Model file for the job. Use its own axes, mm. Face numbers are marked on the shaded views. A direction names the side the tool comes from. Round coordinates to 2 decimals unless told otherwise and drop trailing zeros. Write each loop counter-clockwise with the first axis right and the second up, starting at its lowest first coordinate (ties: lowest second). Pieces come first, ordered by that corner, then holes.
```python
from build123d import *

# Parameters (mm, degrees)
SKETCH1_W           = 7
SKETCH1_H           = 1
BOSS_EXTRUDE1_DEPTH = 3


with BuildPart() as part:
    # Sketch1 → Boss-Extrude1 (new body, symmetric)
    with BuildSketch(Plane(origin=(0, 0, 0), x_dir=(1, 0, 0), z_dir=(0, 1, 0))):
        with Locations((-3.5, 0)):
            Rectangle(SKETCH1_W, SKETCH1_H)
        Polygon((1, 0.5), (0, 0.5), (0, -0.5), (0, -4), (10, -4), (10, -3), (1, -3), align=None)
    extrude(amount=BOSS_EXTRUDE1_DEPTH, both=True)


solid = part.part
```
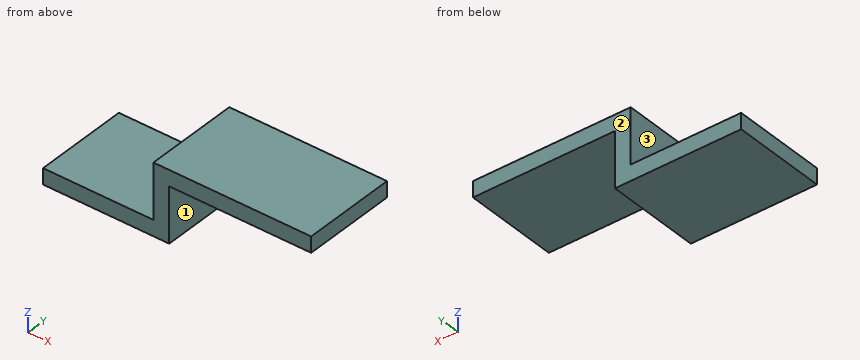
1) Cut at C-C on x = 2.5. List the corners of the cut face in (y, z), and give its area (3 significant figures).
2) Cut at A-A on y = 1.2. List the corners of the cut face in (x, z).
3) Which spindle directions (+Z, -Z, +X, -X, +Y, -Y) get a long thin tool onto all of the face, cutting with end or side? Do the marked faces 1, 2 and 3. Say none if no direction does.
4) Flat gauge pins, fed straight in: pin 1 Ø1.8 at (y, z) = (-0.5, 1) entering from +X; pin 2 Ø1.8 at (y, z) = (0.5, 2.5) entering from -X; pin 3 Ø3 at (x, y) = (6.5, 1.5) entering from -Z. Where does each tip first touch, or does it go through?
5) Cut at B-B on z = 1.75. List the corners of the cut face in (x, y).
6) Wall check: probe 1 along Z at (x, y) = (-5, -2.2); probe 2 along X at (y, z) = (-1.3, 1.75); probe 3 along X at (y, z) = (2.15, 0.1). Give the ranges that are in metal, low to high.
Result sheet:
1. outline: (-3, 3) - (3, 3) - (3, 4) - (-3, 4) - close
1. area: 6.00 mm2
2. outline: (-7, -0.5) - (1, -0.5) - (1, 3) - (10, 3) - (10, 4) - (0, 4) - (0, 0.5) - (-7, 0.5) - close
3. face 1: -Z, +X, +Y, -Y
3. face 2: +Z, -Z, +X, -X, +Y
3. face 3: +Z, -X, +Y, -Y
4. pin 1: stops at x = 1
4. pin 2: stops at x = 0
4. pin 3: stops at z = 3
5. outline: (0, -3) - (1, -3) - (1, 3) - (0, 3) - close
6. probe 1: z = -0.5 to 0.5
6. probe 2: x = 0 to 1
6. probe 3: x = -7 to 1
